Input: part model. Units: mm. Frame: model coordinates. A direction names the side the tool comes from. Give positions to 0.01 mm unless a question says otherwise; leave off trailing zeros. Order: outer loops, then holes, each group sorted by start corner. A loop starts at its lowest first (then second) coordinate and runs counter-clockwise, first axis right, second up. Notation, with made-up numbers: (25, 51) - (41, 51) arc R17 ccw to (41, 80) - close; hole circle Ø1 at (-9, -5). An arc over 180 degrees is marked (long way). Answer in a Markdown table with one row per item. Add a question column.
1. Section query D-D on y = -3.5. Return loops of the section in (x, z).
2. Section query B-B on x = 12. Return loops of the section in (y, z), and give its area (3 significant figures).
3. Mould query, pull axis Y, two halves, no side actions, for faces 1 (the face through (-4, 0, 5)), 2 (the face through (4, -2, 0)), 3 (the face through (7.189, -4.294, 4.93)). Classes: released by +Y, released by -Y, zero draft, split by the parting line, or undercut.
4. Ray query, line 1 (Y direction, x = 12.75, z = 1); line 2 (Z direction, x = 12, y = 2.9); line 3 (Y direction, x = 0, z = 4.5). Return the intervals inside material, ascending. Write a range as [from, to].
5. Contact query for flat-ended pins moving along their axis: pin 1 (5 mm diameter, centred on x = 0, y = 0, fed in from -Z); pin 2 (2 mm diameter, centred on y = -6, z = 1.5, fed in from +X); pin 3 (5 mm diameter, centred on x = 12, z = 5, fed in from -Y); pin 4 (3 mm diameter, centred on x = 8, z = 6.5, fed in from +Y). Output: stop coordinate, or through.
6. Section query C-C on x = 0. Return loops of the section in (y, z).
7. Section query A-A on z = 5. Return loops of the section in (x, y).
8. Access query for faces 4 (the face through (9.85, 1, 4.93)), 5 (the face through (14, 4, 4)), 6 (the face through (16, -3, 5)), 7 (the face through (14, -4, 4)), 8 (the face through (4, -2, 10)). Directions: +Z, -Z, +X, -X, +Y, -Y. A direction counts if a zero-diameter tool reaches every point of the face in a straight line with its end or side. Return the directions, or none.
```python
from build123d import *

# Parameters (mm, degrees)
F1_DEPTH = 10
F2_R     = 2
F3_DEPTH = 12.001


with BuildPart() as f1:
    # F0 (on Top) → F1 (new body)
    with BuildSketch(Plane.XY):
        with BuildLine():
            ThreePointArc((3.872983, -1), (-4, 0), (3.872983, 1))
            Line((3.872983, 1), (16, 1))
            Line((16, 1), (16, 4))
            Line((16, 4), (8.485281, 4))
            ThreePointArc((8.485281, 4), (7.206077, 4.286398), (6.171114, 5.090909))
            ThreePointArc((6.171114, 5.090909), (-8, 0), (6.171114, -5.090909))
            ThreePointArc((6.171114, -5.090909), (7.206077, -4.286398), (8.485281, -4))
            Line((8.485281, -4), (16, -4))
            Line((16, -4), (16, -1))
            Line((16, -1), (3.872983, -1))
        make_face()
    extrude(amount=F1_DEPTH)

    # F2 (on face) → F3 (cut, through all)
    with BuildSketch(Plane.XZ.offset(4)):
        with Locations((12, 5)):
            Circle(F2_R)
    extrude(amount=-F3_DEPTH, mode=Mode.SUBTRACT)


solid = f1.part
```
Answer:
| question | item | result |
|---|---|---|
| 1 | outline | (-7.19, 0) - (-1.94, 0) - (-1.94, 10) - (-7.19, 10) - close; (1.94, 0) - (16, 0) - (16, 10) - (1.94, 10) - close; hole circle Ø4 at (12, 5) |
| 2 | outline | (-4, 0) - (-1, 0) - (-1, 3) - (-4, 3) - close; (-4, 7) - (-1, 7) - (-1, 10) - (-4, 10) - close; (1, 0) - (4, 0) - (4, 3) - (1, 3) - close; (1, 7) - (4, 7) - (4, 10) - (1, 10) - close |
| 2 | area | 36.0 mm² |
| 3 | face 1 | undercut |
| 3 | face 2 | zero draft |
| 3 | face 3 | released by -Y |
| 4 | line 1 | y = [-4, -1], [1, 4] |
| 4 | line 2 | z = [0, 3], [7, 10] |
| 4 | line 3 | y = [-8, -4], [4, 8] |
| 5 | pin 1 | passes through |
| 5 | pin 2 | stops at x = 6.25 |
| 5 | pin 3 | stops at y = -4 |
| 5 | pin 4 | stops at y = 4.75 |
| 6 | outline | (-8, 0) - (-4, 0) - (-4, 10) - (-8, 10) - close; (4, 0) - (8, 0) - (8, 10) - (4, 10) - close |
| 7 | outline | (3.87, -1) arc R4 cw (long way) to (3.87, 1) - (10, 1) - (10, 4) - (8.49, 4) arc R3 cw to (6.17, 5.09) arc R8 ccw (long way) to (6.17, -5.09) arc R3 cw to (8.49, -4) - (10, -4) - (10, -1) - close; (14, -4) - (16, -4) - (16, -1) - (14, -1) - close; (14, 1) - (16, 1) - (16, 4) - (14, 4) - close |
| 8 | face 4 | +Z, -Z, +X |
| 8 | face 5 | +Z, -Z, +X, +Y |
| 8 | face 6 | +Z, -Z, +X, +Y, -Y |
| 8 | face 7 | +Z, -Z, +X, -Y |
| 8 | face 8 | +Z, +X, -X, +Y, -Y |
